Check sheet for the modelled part. Datum: model origin and axes. Units: mm. Face numbers are marked on the shaded views. A direction names the side the tool comes from. Round coordinates to 2 decimals unless told otherwise and drop trailing zeros. Loops run counter-clockwise (first coordinate to the right, second up) from the corner with the lowest first, then second, coordinate; pieces in that order, holes last. Notation, with made-up numbers: (65.25, 13.5) - (117.25, 13.5) arc R20 ccw to (117.25, 35.5) - close; hole circle Ø9 at (41.25, 50). An arc over 180 degrees is marked (long way). Put each result on its own line as item: value. Start each with the question number.
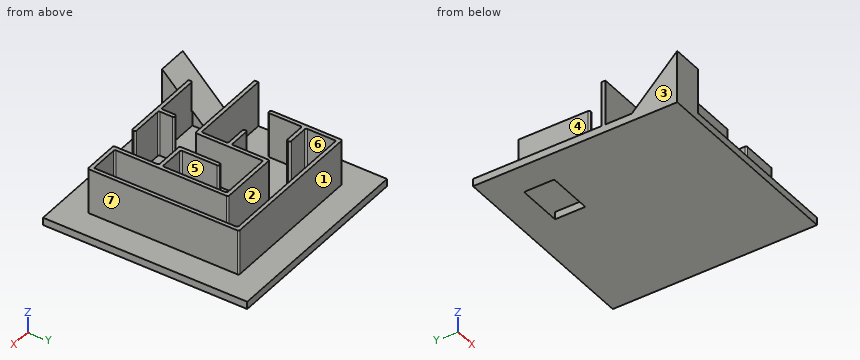
```python
from build123d import *

# Parameters (mm, degrees)
F1_DEPTH = 5
F2_DEPTH = 35
F4_DEPTH = 25
F0_W     = 15
F0_H     = 2.5
F0_W_2   = 2.5
F0_H_2   = 10
F5_DEPTH = 35
F6_R     = 1


# Not quite as in the source:
# - two fillets or chamfers of one size are made in one step


with BuildPart() as f1:
    # F0 (on Top) → F1 (new body)
    with BuildSketch(Plane.XY):
        Polygon((67.5, 67.5), (-67.5, 67.5), (-67.5, -17.5), (-12.5, -17.5), (-12.5, 0), (-27.5, 0), (-27.5, 2.5), (-12.5, 2.5), (-12.5, 25), (-12.5, 27.5), (-10, 27.5), (27.5, 27.5), (27.5, -17.5), (27.5, -20), (27.5, -47.5), (47.5, -47.5), (47.5, 47.5), (-17.5, 47.5), (-17.5, 27.5), (-32.5, 27.5), (-32.5, 25), (-47.5, 25), (-47.5, 2.5), (-50, 2.5), (-50, 50), (50, 50), (50, -50), (25, -50), (25, -20), (5, -20), (5, 7.5), (7.5, 7.5), (7.5, -17.5), (25, -17.5), (25, 25), (-10, 25), (-10, -20), (-67.5, -20), (-67.5, -37.5), (-47.5, -37.5), (-47.5, -47.5), (-17.5, -47.5), (-17.5, -37.5), (-15, -37.5), (-15, -47.5), (7.5, -47.5), (7.5, -50), (-47.5, -50), (-47.5, -67.5), (67.5, -67.5), align=None)
    extrude(amount=F1_DEPTH)

    # F0 (on Top) → F2 (join)
    with BuildSketch(Plane.XY):
        Polygon((-67.5, -67.5), (-47.5, -67.5), (-47.5, -50), (-47.5, -47.5), (-47.5, -37.5), (-67.5, -37.5), align=None)
    extrude(amount=F2_DEPTH)

    # F3 (on face) → F4 (cut)
    with BuildSketch(Plane.YZ.offset(-47.5)):
        Polygon((-37.5, 35), (-67.5, 35), (-37.5, 5), align=None)
    extrude(amount=-F4_DEPTH, mode=Mode.SUBTRACT)

    # F0 (on Top) → F5 (join)
    with BuildSketch(Plane.XY):
        Polygon((27.5, -20), (25, -20), (25, -50), (50, -50), (50, 50), (-50, 50), (-50, 2.5), (-47.5, 2.5), (-47.5, 25), (-47.5, 27.5), (-47.5, 47.5), (-17.5, 47.5), (47.5, 47.5), (47.5, -47.5), (27.5, -47.5), align=None)
        Polygon((-47.5, -47.5), (-47.5, -50), (7.5, -50), (7.5, -47.5), (-15, -47.5), (-17.5, -47.5), align=None)
        Polygon((-12.5, -17.5), (-67.5, -17.5), (-67.5, -20), (-10, -20), (-10, 25), (-12.5, 25), (-12.5, 2.5), (-12.5, 0), align=None)
        with Locations((-20, 1.25)):
            Rectangle(F0_W, F0_H)
        with Locations((-40, 26.25)):
            Rectangle(F0_W, F0_H)
        Polygon((-10, 27.5), (-10, 25), (25, 25), (25, -17.5), (27.5, -17.5), (27.5, 27.5), align=None)
        with Locations((-11.25, 26.25)):
            Rectangle(F0_W_2, F0_H)
        Polygon((25, -20), (25, -17.5), (7.5, -17.5), (7.5, 7.5), (5, 7.5), (5, -20), align=None)
        with Locations((26.25, -18.75)):
            Rectangle(F0_W_2, F0_H)
        with Locations((-16.25, -42.5)):
            Rectangle(F0_W_2, F0_H_2)
    extrude(amount=F5_DEPTH)

    # F6
    f6_edges = [f1.edges().sort_by_distance(p)[0] for p in [
        (7.5, -50, 20),
        (7.5, -47.5, 20),
        (-10, -20, 20),
        (-15, -37.5, 20),
        (5, -20, 20),
        (25, -50, 20),
        (50, -50, 20),
        (27.5, 27.5, 20),
        (50, 50, 20),
        (-47.5, 47.5, 17.5),
        (-27.5, 0, 20),
        (-47.5, 25, 20),
        (-32.5, 25, 20),
        (-32.5, 27.5, 20),
        (-10, 25, 20),
        (7.5, 7.5, 20),
        (-47.5, 2.5, 20),
        (-50, 2.5, 20),
        (-47.5, -47.5, 25),
        (-50, 50, 20),
        (25, -20, 20),
        (-12.5, 2.5, 20),
        (25, -17.5, 20),
        (-12.5, -17.5, 20),
        (27.5, -47.5, 20),
        (-12.5, 27.5, 20),
        (-47.5, 27.5, 17.5),
        (7.5, -17.5, 20),
        (-17.5, -37.5, 20),
        (25, 25, 20),
        (-15, -47.5, 20),
        (-17.5, -47.5, 20),
        (5, 7.5, 20),
        (47.5, 47.5, 20),
        (-27.5, 2.5, 20),
        (-12.5, 0, 20),
    ]]
    fillet(f6_edges, radius=F6_R)


solid = f1.part
```
Q1. Cross-section at C-C on z = 25. State how many separate pieces and enclosed holes the cut face has, and give its area (3 significant figures).
Q2. Cross-section at A-A on x = -44. Enter the section's corners in (y, z).
Q3. Depth check by flat-ended pin: pin 1 Ø12 at (x, y) = (6, -10.5) entering from -Z; pin 2 Ø8 at (x, z) = (19, 13) entering from +Y; pin 3 Ø1 at (y, z) = (13.5, 26) entering from +X; pin 4 Ø1 at (x, y) = (51.5, 9) entering from +Z. Enter the tip coordinate at first touch or a pass-through.
Q4. Cross-section at B-B on y = 20.5. Enter the section's corners in (x, z), and give its area (3 significant figures).
Q5. Material ranges on line 1 (Y direction, x = 14, z = 16); line 2 (Y direction, x = -44, z = 31); line 3 (X direction, y = -10.5, z = 25), recorded low to high. Write a range as from..to.
Q6. Set-up check for the marked faces 4, 5, 6 and 7: record each of +Z, -Z, +X, -X, +Y, -Y from which the full face is reachable in a straight line by a thin tool's end or side.
Q7. Cross-section at D-D on y = -31.5. Enter the section's corners in (x, z).
Q8. Draft check along X on the marked faces 1, 2 and 3. Enter one of: +X half, -X half, draft (parallel to the pull), parting line (faces both ways), or undercut.
Answer list:
1. separate pieces: 3
1. enclosed holes: 0
1. area: 1,740 mm2
2. outline: (-67.5, 0) - (27.5, 0) - (27.5, 35) - (25, 35) - (25, 5) - (-17.5, 5) - (-17.5, 35) - (-20, 35) - (-20, 5) - (-47.5, 5) - (-47.5, 35) - (-50, 35) - (-50, 5) - (-67.5, 5) - close; (47.5, 0) - (67.5, 0) - (67.5, 5) - (50, 5) - (50, 35) - (47.5, 35) - close
3. pin 1: stops at z = 0
3. pin 2: stops at y = 50
3. pin 3: stops at x = 50
3. pin 4: stops at z = 5
4. outline: (-67.5, 0) - (67.5, 0) - (67.5, 5) - (50, 5) - (50, 35) - (47.5, 35) - (47.5, 5) - (27.5, 5) - (27.5, 35) - (25, 35) - (25, 5) - (-10, 5) - (-10, 35) - (-12.5, 35) - (-12.5, 5) - (-47.5, 5) - (-47.5, 35) - (-50, 35) - (-50, 5) - (-67.5, 5) - close
4. area: 975 mm2
5. line 1: y = -20..-17.5, 25..27.5, 47.5..50
5. line 2: y = -50..-47.5, -20..-17.5, 25..27.5, 47.5..50
5. line 3: x = -12.5..-10, 5..7.5, 25..27.5, 47.5..50
6. face 4: +Z, -X, +Y
6. face 5: +Z
6. face 6: +Z, -Z
6. face 7: +Z, +X, +Y, -Y
7. outline: (-67.5, 0) - (67.5, 0) - (67.5, 5) - (50, 5) - (50, 35) - (47.5, 35) - (47.5, 5) - (27.5, 5) - (27.5, 35) - (25, 35) - (25, 5) - (-67.5, 5) - close
8. face 1: draft
8. face 2: undercut
8. face 3: -X half
